Geometry: final body of the model. Coordinates: model frame, mm. A direction names the side the tool comes from. Coordinates: 2 decimals unless noted, no trailing zeros. Loops run counter-clockwise (first coordinate to the right, second up) from the corner with the lowest first, then second, coordinate; pieces in that order, holes last. Notation, with made-up numbers: (27.25, -20) - (53.25, -20) arc R21 cw to (53.25, -16) - close; hole circle Ø10 at (-8.5, -14). An arc over 180 degrees is marked (long way). Return JSON: item names as keys, results as strings.
from build123d import *

# Parameters (mm, degrees)
F0_W     = 5.588
F0_H     = 33.6042
F0_R     = 0.9906
F2_DEPTH = 5.588
F3_W     = 1.4605
F3_H     = 2.5908
F3_H_2   = 2.794
F4_DEPTH = 5.589


# Not quite as in the source:
# - the program builds the solid bodies; features that only make, move or delete a surface that nothing else refers to are left out


with BuildPart() as f2:
    # F0 (on Front) → F2 (new body)
    with BuildSketch(Plane.XZ):
        Rectangle(F0_W, F0_H)
        with BuildLine():
            ThreePointArc((-0.9271, 14.986), (0, 15.9131), (0.9271, 14.986))
            Line((0.9271, 14.986), (0.9271, -14.986))
            ThreePointArc((0.9271, -14.986), (0, -15.9131), (-0.9271, -14.986))
            Line((-0.9271, -14.986), (-0.9271, 14.986))
        make_face(mode=Mode.SUBTRACT)
        with BuildLine():
            Line((-2.794, 16.8021), (2.794, 16.8021))
            Line((2.794, 16.8021), (2.794, 22.3901))
            ThreePointArc((2.794, 22.3901), (0, 25.1841), (-2.794, 22.3901))
            Line((-2.794, 22.3901), (-2.794, 16.8021))
        make_face()
        with Locations((0, 22.3901)):
            Circle(F0_R, mode=Mode.SUBTRACT)
        with BuildLine():
            Line((2.794, -22.3901), (2.794, -16.8021))
            Line((2.794, -16.8021), (-2.794, -16.8021))
            Line((-2.794, -16.8021), (-2.794, -22.3901))
            ThreePointArc((-2.794, -22.3901), (0, -25.1841), (2.794, -22.3901))
        make_face()
        with Locations((0, -22.3901)):
            Circle(F0_R, mode=Mode.SUBTRACT)
    extrude(amount=F2_DEPTH)

    # F3 (on face) → F4 (cut, through all)
    with BuildSketch(Plane(origin=(-2.794, 0, 0), x_dir=(0, -1, 0), z_dir=(-1, 0, 0))):
        with Locations((0.73025, 21.0947)):
            Rectangle(F3_W, F3_H)
        with Locations((0.73025, 23.7871)):
            Rectangle(F3_W, F3_H_2)
        with Locations((4.85775, 23.7871)):
            Rectangle(F3_W, F3_H_2)
        with Locations((4.85775, 21.0947)):
            Rectangle(F3_W, F3_H)
    extrude(amount=-F4_DEPTH, mode=Mode.SUBTRACT)


solid = f2.part
Item 1: Reachability of faces 5 (the face through (0.02, -2.755, -15.913)), 6 (the face through (0, -1, 19.799)), 7 (the face through (0, -4.128, 21)) from +Z, -Z, +X, -X, +Y, -Y: full face, straight path, thin tool, end or side. Return the list, or none.
Worked out:
{"face 5": "+Y, -Y", "face 6": "+Z, +X, -X, +Y", "face 7": "+Z, +X, -X, -Y"}
Item 2: Ray query, probe 1 along Z at (x, y) = (0, -2.4); probe 2 along Z at (x, y) = (0, -4.35); probe 3 along X at (y, z) = (-5.2, 10). Return the intervals inside material, ascending. Write a range as from..to.
Worked out:
{"probe 1": "-25.18..-23.38, -21.4..-15.91, 15.91..21.4, 23.38..25.18", "probe 2": "-25.18..-23.38, -21.4..-15.91, 15.91..19.8", "probe 3": "-2.79..-0.93, 0.93..2.79"}
Item 3: Section query C-C, the plane x = 0. Return loops of the section in (y, z).
Worked out:
{"outline": "(-5.59, -25.18) - (0, -25.18) - (0, -23.38) - (-5.59, -23.38) - close; (-5.59, -21.4) - (0, -21.4) - (0, -15.91) - (-5.59, -15.91) - close; (-5.59, 15.91) - (0, 15.91) - (0, 19.8) - (-1.46, 19.8) - (-1.46, 21.4) - (-4.13, 21.4) - (-4.13, 19.8) - (-5.59, 19.8) - close; (-4.13, 23.38) - (-1.46, 23.38) - (-1.46, 25.18) - (-4.13, 25.18) - close"}
Item 4: Section query D-D, the plane y = -2.1. Return loops of the section in (x, z).
Worked out:
{"outline": "(-2.79, -22.39) arc R2.79 ccw to (2.79, -22.39) - (2.79, 22.39) arc R2.79 ccw to (-2.79, 22.39) - close; hole circle Ø1.98 at (0, -22.39); hole circle Ø1.98 at (0, 22.39); hole (-0.93, -14.99) arc R0.93 ccw to (0.93, -14.99) - (0.93, 14.99) arc R0.93 ccw to (-0.93, 14.99) - close"}
Item 5: Section query B-B, the plane y = -5.15. Return loops of the section in (x, z).
Worked out:
{"outline": "(-2.79, -22.39) arc R2.79 ccw to (2.79, -22.39) - (2.79, 19.8) - (-2.79, 19.8) - close; hole circle Ø1.98 at (0, -22.39); hole (-0.93, -14.99) arc R0.93 ccw to (0.93, -14.99) - (0.93, 14.99) arc R0.93 ccw to (-0.93, 14.99) - close"}
Item 6: First-contact query: pin 1 Ø1.6 at (x, z) = (0, 21.5) entering from +Y; pin 2 Ø1.5 at (x, y) = (1.5, -1) entering from +Z; pin 3 Ø3 at (x, z) = (0, 22.39) entering from -Y; pin 4 Ø1.2 at (x, z) = (0, -22.39) entering from -Y. Flat tips, straight axial feed; report the tip coordinate or a pass-through.
Worked out:
{"pin 1": "y = -1.46", "pin 2": "z = 25.03", "pin 3": "y = -4.13", "pin 4": "through"}
Item 7: Mould query, pull axis X, two halves, no side actions, for faces 1 (the face through (1.2, -5.588, -2.4)), 2 (the face through (2.794, -3, 0)), 3 (the face through (-0.02, -2.755, 15.913)), 4 (the face through (0.927, -3, 0)). Classes: +X half, -X half, draft (parallel to the pull), parting line (faces both ways), or undercut.
Worked out:
{"face 1": "draft", "face 2": "+X half", "face 3": "undercut", "face 4": "undercut"}
Item 8: Section query A-A, the plane z = 14. Return loops of the section in (x, y), and give its area (3 significant figures).
Worked out:
{"outline": "(-2.79, -5.59) - (-0.93, -5.59) - (-0.93, 0) - (-2.79, 0) - close; (0.93, -5.59) - (2.79, -5.59) - (2.79, 0) - (0.93, 0) - close", "area": "20.9 mm^2"}
